```python
from build123d import *

# Parameters (mm, degrees)
SKETCH1_R           = 6.5
BOSS_EXTRUDE1_DEPTH = 12
BOSS_EXTRUDE2_DEPTH = 5
BOSS_EXTRUDE3_DEPTH = 23
SKETCH4_R           = 3.5
CUT_EXTRUDE1_DEPTH  = 42.443459209


with BuildPart() as part:
    # Sketch1 → Boss-Extrude1 (new body)
    with BuildSketch(Plane.XY):
        Circle(SKETCH1_R)
    extrude(amount=BOSS_EXTRUDE1_DEPTH)

    # Sketch2 → Boss-Extrude2 (add)
    with BuildSketch(Plane(origin=(0, 0, 0), x_dir=(-1, 0, 0), z_dir=(0, 0, -1))):
        Polygon((-7.393524213, -3.055454092), (-1.050661243, -7.930706838), (6.342862971, -4.875252746), (7.393524213, 3.055454092), (1.050661243, 7.930706838), (-6.342862971, 4.875252746), align=None)
    extrude(amount=BOSS_EXTRUDE2_DEPTH)

    # Sketch3 → Boss-Extrude3 (add)
    with BuildSketch(Plane(origin=(0, 0, -5), x_dir=(-1, 0, 0), z_dir=(0, 0, -1))):
        with BuildLine():
            ThreePointArc((4.620952633, 1.909658808), (-1.909658808, 4.620952633), (-4.620952633, -1.909658808))
            Line((-4.620952633, -1.909658808), (4.620952633, 1.909658808))
        make_face()
        with BuildLine():
            Line((4.620952633, 1.909658808), (-4.620952633, -1.909658808))
            ThreePointArc((-4.620952633, -1.909658808), (0.973456941, -4.904322745), (5, 0))
            ThreePointArc((5, 0), (4.904322745, 0.973456941), (4.620952633, 1.909658808))
        make_face()
    extrude(amount=BOSS_EXTRUDE3_DEPTH)

    # Sketch4 → Cut-Extrude1 (cut, through all)
    with BuildSketch(Plane.XY.offset(12)):
        Circle(SKETCH4_R)
    extrude(amount=-CUT_EXTRUDE1_DEPTH, mode=Mode.SUBTRACT)


solid = part.part
```
CAD build for the part. Positions are in the model's coordinates, mm. A direction names the side the tool comes from. Round coordinates to 2 decimals unless told otherwise and drop trailing zeros. Write each loop counter-clockwise with the first axis right and the second up, starting at its lowest first coordinate (ties: lowest second). Pieces come first, ordered by that corner, then holes.
Item 1: Band-saw the part on B-B on z = 8. Write the cut outline in (x, y), then the cut area to 3 significant figures.
Filled in:
outline: circle Ø13 at (0, 0); hole circle Ø7 at (0, 0)
area: 94.2 mm2
Item 2: Tool access for faces 1 (the flat face through (-2.594, -6.424, -2.465)), 2 (the flat face through (3, 6, 0)): list every direction of +Z, -Z, +X, -X, +Y, -Y with a clear straight run to the whole face (end or side of a thin tool).
Filled in:
face 1: +Z, -Z, -X, -Y
face 2: +Z
Item 3: Band-saw the part on C-C on x = 4. Write the cut outline in (y, z).
Filled in:
outline: (-5.66, -5) - (-3, -5) - (-3, -28) - (3, -28) - (3, -5) - (5.84, -5) - (5.84, 0) - (5.12, 0) - (5.12, 12) - (-5.12, 12) - (-5.12, 0) - (-5.66, 0) - close
Item 4: Band-saw the part on A-A on x = 2. Write the cut outline in (y, z).
Filled in:
outline: (-7.2, -5) - (-4.58, -5) - (-4.58, -28) - (-2.87, -28) - (-2.87, 12) - (-6.18, 12) - (-6.18, 0) - (-7.2, 0) - close; (2.87, -28) - (4.58, -28) - (4.58, -5) - (6.67, -5) - (6.67, 0) - (6.18, 0) - (6.18, 12) - (2.87, 12) - close
Item 5: Mould opens along X. For faces 3 (the cylindrical face through (3.233, -1.341, -7.72)), 4 (the flat face through (2.594, 6.424, -2.465)), 5 (the flat face through (-5, -2, -5)), 6 (the flat face through (-4.266, 5.459, -2.465)) say: released by +X, released by -X, zero draft, split by the parting line, or undercut.
Filled in:
face 3: undercut
face 4: released by +X
face 5: zero draft
face 6: released by -X
Item 6: Drop flat-ended pins along their axis: pin 1 Ø6.5 at (x, y) = (0, 0) entering from -Z; pin 2 Ø4 at (y, z) = (5.5, -4.5) entering from -X; pin 3 Ø2 at (y, z) = (0.5, -23.5) entering from +X; pin 4 Ø6 at (y, z) = (4.5, 5) entering from -X. Give the stop position or say it passes through.
Filled in:
pin 1: passes through
pin 2: stops at x = -6.82
pin 3: stops at x = 5
pin 4: stops at x = -6.32
Item 7: Drill centre lines: L1, parallel to Y at x = 0, z = -15; L2, parallel to Y at x = -2.75, z = -17; L3, parallel to Z at x = -0.75, y = 6. Where is each one in solid material? Low to high.
Filled in:
L1: y = -5 to -3.5, 3.5 to 5
L2: y = -4.18 to -2.17, 2.17 to 4.18
L3: z = -5 to 12
Item 8: Band-saw the part on D-D on y = 4. Write the cut outline in (x, z), then the cut area to 3 significant figures.
Filled in:
outline: (-6.16, -5) - (-3, -5) - (-3, -28) - (3, -28) - (3, -5) - (6.46, -5) - (6.46, 0) - (5.12, 0) - (5.12, 12) - (-5.12, 12) - (-5.12, 0) - (-6.16, 0) - close
area: 324 mm2
